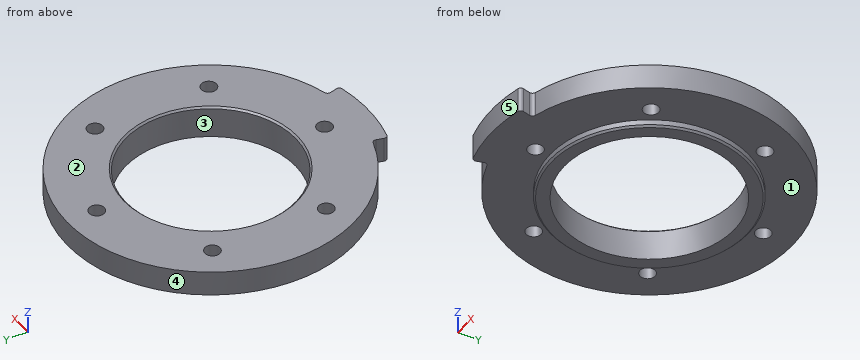
Autodesk Inventor part; units mm, degrees
ref_plane "YZ Plane" through (0, 0, 0) normal (1, 0, 0) x (0, 1, 0)
ref_plane "XZ Plane" through (0, 0, 0) normal (0, 1, 0) x (-1, 0, 0)
ref_plane "XY Plane" through (0, 0, 0) normal (0, 0, 1) x (1, 0, 0)
sketch "スケッチ2" plane through (0, 0, 0) normal (1, 0, 0) x (0, 1, 0)
  line L0 (24, 0) -> (24, -9)
  line L1 (40.5, 0) -> (40.5, -7)
  line L2 (40.5, 0) -> (24, 0)
  line L3 (24, 0) -> (59, 0)
  line L4 (24, -9) -> (28, -9)
  line L5 (0, -10.8) -> (0, 1.8)
  line L6 (28, -9) -> (28, -7)
  line L7 (28, -7) -> (40.5, -7)
  point P0 (0, 0)
  dimension "d40" = 24
  dimension "d41" = 7
  dimension "d42" = 40.5
  dimension "d43" = 28
  dimension "d44" = 2
revolve "回転1" add sketch "スケッチ2" angle 360 about axis through (0, 0, -10) along (0, 0, 1)
sketch "スケッチ4" plane through (0, 0, 0) normal (0, 0, 1) x (1, 0, 0)
  point P0 (0, 0)
  point P1 (0, 32)
  point P2 (-27.7128, 16)
  point P3 (-27.7128, -16)
  point P4 (0, -32)
  point P5 (27.7128, -16)
  point P6 (27.7128, 16)
  dimension "d11" = 32
  dimension "d14" = 360
hole "穴1" at (0, 32, 0) at (-27.7128, 16, 0) at (-27.7128, -16, 0) at (0, -32, 0) at (27.7128, -16, 0) at (27.7128, 16, 0) direction (0, 0, -1) diameter 4.3 end through all
chamfer "面取り3" distance 0.5 angle 45 1 edges at (0, -28, -9)
chamfer "面取り4" distance 0.5 angle 45 1 edges at (0, -24, 0)
sketch "スケッチ7" plane through (0, 0, 0) normal (0, 0, 1) x (1, 0, 0)
  circle A0 centre (0, 0) radius 40.5
  circle A1 centre (0, 0) radius 44.5
  line L0 (0, 0) -> (11.5174, -42.9837)
  line L1 (0, 0) -> (-11.5174, -42.9837)
  line L2 (0, 62.3) -> (0, -62.3)
  point P0 (10.4822, -39.12)
  point P1 (-10.4822, -39.12)
  dimension "d51" = 4
  dimension "d52" = 15
  dimension "d53" = 15
extrude "押し出し3" add sketch "スケッチ7" against normal up to surface (7 mm away) contours L0 A1 L2 A0 | A0 L2 A1 L1 picked at (6.2128, -42.6798) picked at (-1.2928, -43.1102)
fillet "フィレット1" radius 1 4 edges at (10.4822, -39.12, -3.5) (11.5174, -42.9837, -3.5) (-10.4822, -39.12, -3.5) (-11.5174, -42.9837, -3.5)
properties part number "base12" material "ABS プラスチック"
Build history of the part. All positions in model axes, mm. Face numbers are marked on the shaded views. A direction names the side the tool comes from. Give positions to 0.01 mm unless a question says otherwise; leave off trailing zeros. Loops run counter-clockwise (first coordinate to the right, second up) from the corner with the lowest first, then second, coordinate; pieces in that order, holes last.
Item 1: Flat gauge pins, fed straight in: pin 1 (12 mm diameter, centred on x = 13.5, y = -33, fed in from -Z); pin 2 (5 mm diameter, centred on y = -4.5, z = -3.5, fed in from -X); pin 3 (4 mm diameter, centred on x = -27.71, y = 16, fed in from +Z); pin 4 (2 mm diameter, centred on y = 24.5, z = -4.5, fed in from +X). Where does each tip first touch, or does it go through?
Answers follow:
pin 1: stops at z = -7
pin 2: stops at x = -40.45
pin 3: passes through
pin 4: stops at x = 32.98
Item 2: Pull direction Y, two halves, no side cores. Call the marked faces 3, 4 and 5: released by +Y, released by -Y, zero draft, split by the parting line, or undercut.
Answers follow:
face 3: undercut
face 4: split by the parting line
face 5: released by -Y
Item 3: Slice it at B-B, the plane z = -1.5. List the corners of the cut face in (x, y).
Answers follow:
outline: (-11.42, -38.86) arc R1 cw to (-10.74, -40.07) - (-11.26, -42.01) arc R1 ccw to (-10.53, -43.24) arc R44.5 ccw to (10.53, -43.24) arc R1 ccw to (11.26, -42.01) - (10.74, -40.07) arc R1 cw to (11.42, -38.86) arc R40.5 ccw (long way) to start; hole circle Ø4.3 at (-27.71, -16); hole circle Ø4.3 at (-27.71, 16); hole circle Ø48 at (0, 0); hole circle Ø4.3 at (0, -32); hole circle Ø4.3 at (0, 32); hole circle Ø4.3 at (27.71, -16); hole circle Ø4.3 at (27.71, 16)
Item 4: Slice it at C-C, the plane y = -16. Give the number of separate pieces and of enclosed holes in the cut face, and give its area (3 significant figures).
Answers follow:
separate pieces: 4
enclosed holes: 0
area: 230 mm2
Item 5: Slice it at A-A, the plane x = 0. List the corners of the cut face in (y, z), and give its area (3 significant figures).
Answers follow:
outline: (-44.5, -7) - (-34.15, -7) - (-34.15, 0) - (-44.5, 0) - close; (-29.85, -7) - (-28, -7) - (-28, -8.5) - (-27.5, -9) - (-24, -9) - (-24, -0.5) - (-24.5, 0) - (-29.85, 0) - close; (24, -9) - (27.5, -9) - (28, -8.5) - (28, -7) - (29.85, -7) - (29.85, 0) - (24.5, 0) - (24, -0.5) - close; (34.15, -7) - (40.5, -7) - (40.5, 0) - (34.15, 0) - close
area: 214 mm2
Item 6: Drill centre lines: line 1 (Y direction, x = 0, z = -1.75); line 2 (X direction, y = 16, z = -4.5); line 3 (X direction, y = -15, z = -0.5) (3 decimals). Where is each one in solid material? Low to high.
Answers follow:
line 1: y = -44.5 to -34.15, -29.85 to -24, 24 to 29.85, 34.15 to 40.5
line 2: x = -37.21 to -29.86, -25.56 to -17.89, 17.89 to 25.56, 29.86 to 37.21
line 3: x = -37.62 to -29.616, -25.81 to -18.735, 18.735 to 25.81, 29.616 to 37.62
Item 7: Which spindle directions (+Z, -Z, +X, -X, +Y, -Y) get a long thin tool onto all of the face, cutting with end or side? Do the marked faces 1 and 2. Say none if no direction does.
Answers follow:
face 1: -Z
face 2: +Z, +X, -X, +Y, -Y
